from build123d import *

# Parameters (mm, degrees)
SKETCH1_R              = 22
BOSS_EXTRUDE1_DEPTH    = 3
SKETCH2_R              = 20
BOSS_EXTRUDE2_DEPTH    = 10
SKETCH3_R              = 25
BOSS_EXTRUDE3_DEPTH    = 3
SKETCH4_R              = 24
BOSS_EXTRUDE4_DEPTH    = 6
SKETCH5_R              = 25
BOSS_EXTRUDE5_DEPTH    = 3
CUT_EXTRUDE1_START     = -3
SKETCH6_R              = 22
SKETCH6_R_2            = 16
CUT_EXTRUDE1_DEPTH     = 3
SKETCH8_R              = 7
CUT_EXTRUDE2_DEPTH     = 2
M12_TAPPED_HOLE1_D     = 10.2
M12_TAPPED_HOLE1_DEPTH = 19


with BuildPart() as part:
    # Sketch1 → Boss-Extrude1 (new body)
    with BuildSketch(Plane.XY):
        Circle(SKETCH1_R)
    extrude(amount=BOSS_EXTRUDE1_DEPTH)

    # Sketch2 → Boss-Extrude2 (add)
    with BuildSketch(Plane.XY.offset(3)):
        Circle(SKETCH2_R)
    extrude(amount=BOSS_EXTRUDE2_DEPTH)

    # Sketch3 → Boss-Extrude3 (add)
    with BuildSketch(Plane.XY.offset(13)):
        Circle(SKETCH3_R)
    extrude(amount=BOSS_EXTRUDE3_DEPTH)

    # Sketch4 → Boss-Extrude4 (add)
    with BuildSketch(Plane.XY.offset(16)):
        Circle(SKETCH4_R)
    extrude(amount=BOSS_EXTRUDE4_DEPTH)

    # Sketch5 → Boss-Extrude5 (add)
    with BuildSketch(Plane.XY.offset(22)):
        Circle(SKETCH5_R)
    extrude(amount=BOSS_EXTRUDE5_DEPTH)

    # Sketch6 → Cut-Extrude1 (cut)
    with BuildSketch(Plane.XY.offset(25).offset(CUT_EXTRUDE1_START)):
        Circle(SKETCH6_R)
        Circle(SKETCH6_R_2, mode=Mode.SUBTRACT)
    extrude(amount=CUT_EXTRUDE1_DEPTH, mode=Mode.SUBTRACT)

    # Sketch8 → Cut-Extrude2 (cut)
    with BuildSketch(Plane.XY.offset(4)):
        Circle(SKETCH8_R)
    extrude(amount=CUT_EXTRUDE2_DEPTH, mode=Mode.SUBTRACT)

    # M12 Tapped Hole1
    with Locations(Plane.XY.offset(25)):
        with Locations((0, 0)):
            Hole(M12_TAPPED_HOLE1_D / 2, depth=M12_TAPPED_HOLE1_DEPTH)


solid = part.part
Source: CAD feature listing. Evaluate the final solid. Frame: model axes, mm. A direction names the side the tool comes from. Round coordinates to 2 decimals unless told otherwise and drop trailing zeros. Loops run counter-clockwise (first coordinate to the right, second up) from the corner with the lowest first, then second, coordinate; pieces in that order, holes last. Notation, with made-up numbers: (25, 17) - (54, 17) arc R36 ccw to (54, 54) - close; hole circle Ø10 at (45.25, -23.75). An arc over 180 degrees is marked (long way). Write item = value, one per line. Start each with the question number.
Item 1: Reachability of faces 1 (the face through (0, 0, 4)), 2 (the face through (-4.769, -21.477, 1.479)), 3 (the face through (1.5, -16.2, 22)) from +Z, -Z, +X, -X, +Y, -Y: full face, straight path, thin tool, end or side. Return the list, or none.
Item 2: Section query D-D on x = 8. Output: boundary loops of the cut face in (y, z).
Item 3: Section query C-C on z = 13.75. Output: boundary loops of the cut face in (x, y).
Item 4: Section query B-B on y = -21. Output: boundary loops of the cut face in (x, z), plus the area to 3 significant figures.
Item 5: Mould query, pull axis Y, two halves, no side actions, for faces 4 (the face through (-9.4, 22.3, 22)), 5 (the face through (-3.47, -15.62, 23.48)), 6 (the face through (23.846, 7.509, 14.479)), 7 (the face through (-5, -2, 6)). Classes: released by +Y, released by -Y, zero draft, split by the parting line, or undercut.
Item 6: Material intervals for line 1 (Y direction, x = 0, z = 4.7); line 2 (Y direction, x = 0, z = 23.7); line 3 (X direction, y = -11, z = 24), sorted ascending.
Item 7: First-contact query: pin 1 Ø7 at (x, y) = (2, -3.5) entering from -Z; pin 2 Ø1.5 at (x, z) = (10.5, 15) entering from +Y; pin 3 Ø6 at (y, z) = (16.5, 17.5) entering from -X; pin 4 Ø6 at (y, z) = (16, 14.5) entering from -X. Flat tips, straight axial feed; report the tip coordinate or a pass-through.
Results list:
q1.face_1 = none
q1.face_2 = -Z
q1.face_3 = +Z
q2.outline = (-23.69, 13) - (-18.33, 13) - (-18.33, 3) - (-20.49, 3) - (-20.49, 0) - (20.49, 0) - (20.49, 3) - (18.33, 3) - (18.33, 13) - (23.69, 13) - (23.69, 16) - (22.63, 16) - (22.63, 22) - (23.69, 22) - (23.69, 25) - (20.49, 25) - (20.49, 22) - (13.86, 22) - (13.86, 25) - (-13.86, 25) - (-13.86, 22) - (-20.49, 22) - (-20.49, 25) - (-23.69, 25) - (-23.69, 22) - (-22.63, 22) - (-22.63, 16) - (-23.69, 16) - close
q3.outline = circle Ø50 at (0, 0); hole circle Ø10.2 at (0, 0)
q4.outline = (-13.56, 13) - (13.56, 13) - (13.56, 16) - (11.62, 16) - (11.62, 22) - (13.56, 22) - (13.56, 25) - (6.56, 25) - (6.56, 22) - (-6.56, 22) - (-6.56, 25) - (-13.56, 25) - (-13.56, 22) - (-11.62, 22) - (-11.62, 16) - (-13.56, 16) - close; (-6.56, 0) - (6.56, 0) - (6.56, 3) - (-6.56, 3) - close
q4.area = 302 mm²
q5.face_4 = zero draft
q5.face_5 = undercut
q5.face_6 = split by the parting line
q5.face_7 = undercut
q6.line_1 = -20 to -7, 7 to 20
q6.line_2 = -25 to -22, -16 to -5.1, 5.1 to 16, 22 to 25
q6.line_3 = -22.45 to -19.05, -11.62 to 11.62, 19.05 to 22.45
q7.pin_1 = 0
q7.pin_2 = 23.02
q7.pin_3 = -20.78
q7.pin_4 = -21.35
